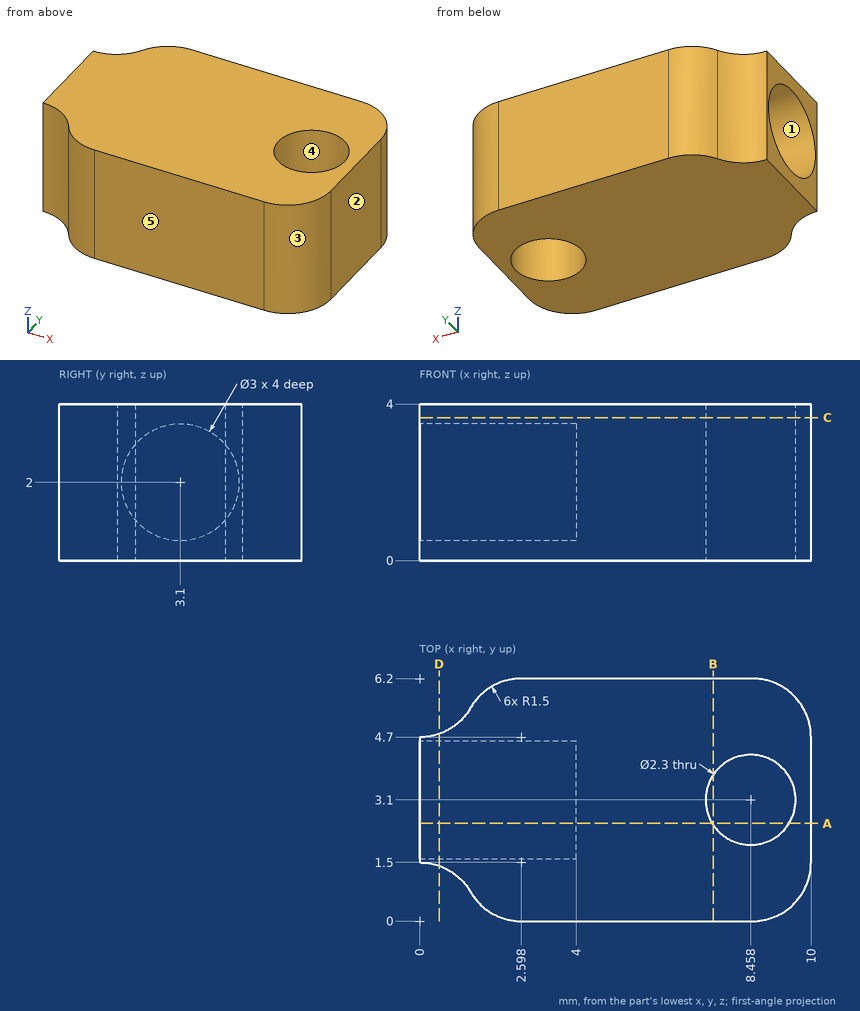
Part print with two shaded views. Sizes in mm from the minimum x, y, z corner. A direction names the side the tool comes from. Round coordinates to 2 decimals unless told otherwise and drop trailing zeros. Write each loop counter-clockwise with the first axis right and the second up, starting at its lowest first coordinate (ties: lowest second). Pieces come first, ordered by that corner, then holes. Notation, with made-up numbers: M 19,5 L 78,5 A17 cw 78,34 Z; hole C 68,-11 d3. An arc over 180 degrees is marked long. Put each result on its own line as item: value. Start each with the question number.
1) 3-axis set-ups, long thin cutter, end or side, ignore diameter. For the marked faces 1 and 2: which of +Z, -Z, +X, -X, +Y, -Y reach the whole face in a straight line?
2) Saw through at A-A, the plane y = 2.5. Write the cut outline in (x, z) (1 decimal).
3) Pull direction X, two halves, no side cores. Call the marked faces 3, 4 and 5: pulls with the +X half, pulls with the -X half, needs draft (parallel to the pull), parting line crosses it, or undercut.
4) Saw through at C-C, the plane z = 3.65. Write the cut outline in (x, y).
5) Drill centre lines: probe 1 along X at (y, z) = (1.75, 2.15); probe 2 along Y at (x, z) = (3, 3); probe 3 along Z at (x, y) = (1.9, 3.1). Where is each one in solid material? Low to high. Write a range as [from, to].
6) Saw through at D-D, the plane x = 0.5. Write the cut outline in (y, z).
7) Saw through at B-B, the plane x = 7.5. Write the cut outline in (y, z), and give its area (3 significant figures).
8) Pin check, flat tip, straight feed: pin 1 Ø1.8 at (x, y) = (8.46, 3.1) entering from -Z. Stop position of the tip, or through.
Resolved:
1. face 1: -X
1. face 2: +Z, -Z, +X, +Y, -Y
2. outline: M 0,0 L 7.5,0 L 7.5,4 L 0,4 L 0,3.4 L 4,3.4 L 4,0.6 L 0,0.6 Z; M 9.4,0 L 10,0 L 10,4 L 9.4,4 Z
3. face 3: pulls with the +X half
3. face 4: undercut
3. face 5: needs draft
4. outline: M 0,1.5 A1.5 cw 1.3,0.75 A1.5 ccw 2.6,0 L 8.5,0 A1.5 ccw 10,1.5 L 10,4.7 A1.5 ccw 8.5,6.2 L 2.6,6.2 A1.5 ccw 1.3,5.45 A1.5 cw 0,4.7 Z; hole C 8.46,3.1 d2.3
5. probe 1: [4, 10]
5. probe 2: [0, 1.98], [4.22, 6.2]
5. probe 3: [0, 0.5], [3.5, 4]
6. outline: M 1.41,0 L 4.79,0 L 4.79,4 L 1.41,4 Z; hole C 3.1,2 d3
7. outline: M 0,0 L 2.46,0 L 2.46,4 L 0,4 Z; M 3.74,0 L 6.2,0 L 6.2,4 L 3.74,4 Z
7. area: 19.7 mm²
8. pin 1: through
